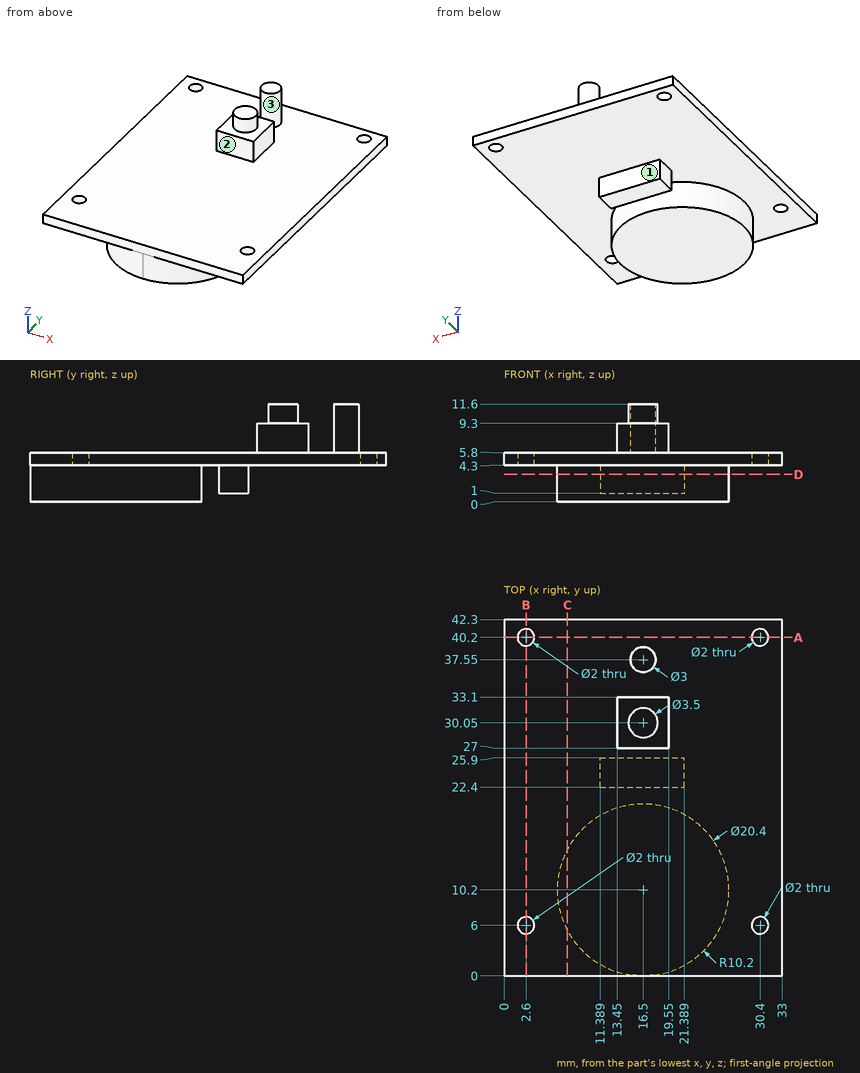
Geometry check sheet. Reference: drawing and pictorial views, mm from the part's lowest x, y, z. Round coordinates to 2 decimals unless told otherwise and drop trailing zeros. Loops run counter-clockwise (first coordinate to the right, second up) from the corner with the lowest first, then second, coordinate; pieces in that order, holes last. Notation, with made-up numbers: M -25.75,23 L -1.75,23 A23 cw -1.75,46 Z; hole C 85.5,40 d7. An arc over 180 degrees is marked long. Return JSON: item names as keys, results as strings. Group by question number.
(1) Scan lines: line 1 along Y through (x, z) = (2.6, 5.2); line 2 along Y through (x, z) = (16.5, 10.25); line 3 along Z through (x, y) = (16, 35). Record each from-to range of solid material in increasing order. Write a range as [from, to].
(2) Section check A-A, the plane y = 40.2. Enter the section's corners in (x, z).
(3) Section check B-B, the plane x = 2.6. Enter the section's corners in (y, z).
(4) Go/stop test with flat-tipped pins: pin 1 (2.5 mm diameter, centred on x = 17, z = 2.5, fed in from +Y); pin 2 (2.5 mm diameter, centred on x = 30.4, y = 40.2, fed in from +Z); pin 3 (1.1 mm diameter, centred on x = 17, z = 7.5, fed in from -Y). Record where each tip stops, or that it passes through.
(5) Mould release check, pull along Y, two halves, no side actions. Record for the marked faces 1, 2 and 3: pulls with the +Y half, pulls with the -Y half, needs draft (parallel to the pull), parting line crosses it, or undercut.
(6) Section check D-D, the plane z = 3.25. Enter the section's corners in (x, y).
(7) Section check C-C, the plane x = 7.5. Enter the section's corners in (y, z), and give its area (3 significant figures).
Data:
{
 "1": {"line 1": "[0, 5], [7, 39.2], [41.2, 42.3]", "line 2": "[28.3, 31.8], [36.05, 39.05]", "line 3": "[4.3, 5.8]"},
 "2": {"outline": "M 0,4.3 L 1.6,4.3 L 1.6,5.8 L 0,5.8 Z; M 3.6,4.3 L 29.4,4.3 L 29.4,5.8 L 3.6,5.8 Z; M 31.4,4.3 L 33,4.3 L 33,5.8 L 31.4,5.8 Z"},
 "3": {"outline": "M 0,4.3 L 5,4.3 L 5,5.8 L 0,5.8 Z; M 7,4.3 L 39.2,4.3 L 39.2,5.8 L 7,5.8 Z; M 41.2,4.3 L 42.3,4.3 L 42.3,5.8 L 41.2,5.8 Z"},
 "4": {"pin 1": "y = 25.9", "pin 2": "z = 5.8", "pin 3": "y = 27"},
 "5": {"face 1": "pulls with the +Y half", "face 2": "pulls with the -Y half", "face 3": "undercut"},
 "6": {"outline": "C 16.5,10.2 d20.4; M 11.39,22.4 L 21.39,22.4 L 21.39,25.9 L 11.39,25.9 Z"},
 "7": {"outline": "M 0,4.3 L 5.4,4.3 L 5.4,0 L 15,0 L 15,4.3 L 42.3,4.3 L 42.3,5.8 L 0,5.8 Z", "area": "105 mm²"}
}
